Can you work these out from the model? Positions are in its coordinate system, mm. A direction names the side the tool comes from. Coordinates: 2 decimals unless noted, no trailing zeros. Write each loop counter-clockwise with the first axis right and the second up, starting at its lowest first coordinate (ties: lowest second). Pieces come first, ordered by that corner, then holes. Notation, with made-up numbers: M 70,60 L 122,60 A15 cw 122,79 Z; hole C 5,-23.75 d10. An arc over 180 degrees is marked long. Use one line per item in the form item = value. Start each with the question number.
```python
from build123d import *

# Parameters (mm, degrees)
SKETCH1_R           = 8.7376
BOSS_EXTRUDE1_DEPTH = 45.085
BOSS_EXTRUDE3_DEPTH = 4.516000112
FILLET2_R           = 5
BOSS_EXTRUDE4_START = 6.096
BOSS_EXTRUDE4_DEPTH = 6.096
CUT_EXTRUDE8_DEPTH  = 6.096
CUT_EXTRUDE10_DEPTH = 12.192
SKETCH23_R          = 1.5875
CUT_EXTRUDE11_DEPTH = 58.161632016
SKETCH24_R          = 3.175
SKETCH24_R_2        = 1.5875
CUT_EXTRUDE12_DEPTH = 54.671581882
CUT_EXTRUDE13_START = -1.27
SKETCH24_2_R        = 3.175
SKETCH24_2_R_2      = 1.5875
CUT_EXTRUDE13_DEPTH = 1.27
FILLET11_R          = 1.778
SKETCH25_R          = 2.5527
CUT_EXTRUDE14_DEPTH = 60.13111817


with BuildPart() as part:
    # Sketch1 → Boss-Extrude1 (new body)
    with BuildSketch(Plane.YZ):
        with Locations(Location((0, 0, 0), (0, 0, 270))):
            Circle(SKETCH1_R)
    extrude(amount=BOSS_EXTRUDE1_DEPTH)

    # Sketch10 → Boss-Extrude3 (add)
    with BuildSketch(Plane(origin=(0, 0, 0), x_dir=(0, -1, 0), z_dir=(-1, 0, 0))):
        with BuildLine():
            Line((0, 8.7376), (34.036, 8.7376))
            Line((34.036, 8.7376), (34.036, -8.7376))
            Line((34.036, -8.7376), (0, -8.7376))
            ThreePointArc((0, -8.7376), (8.7376, 0), (0, 8.7376))
        make_face()
    extrude(amount=-BOSS_EXTRUDE3_DEPTH)

    # Fillet2
    fillet2_edges = [part.edges().sort_by_distance(p)[0] for p in [
        (2.258000056, -34.036, 8.7376),
        (2.258000056, -34.036, -8.7376),
    ]]
    fillet(fillet2_edges, radius=FILLET2_R)

    # Sketch15 → Boss-Extrude4 (add)
    with BuildSketch(Plane.YZ.offset(4.516000112).offset(BOSS_EXTRUDE4_START)):
        with BuildLine():
            Line((-20.066, 5.472786999), (-29.036, 8.7376))
            ThreePointArc((-29.036, 8.7376), (-32.571533906, 7.273133906), (-34.036, 3.7376))
            Line((-34.036, 3.7376), (-34.036, -3.7376))
            ThreePointArc((-34.036, -3.7376), (-32.571533906, -7.273133906), (-29.036, -8.7376))
            Line((-29.036, -8.7376), (-20.066, -8.7376))
            Line((-20.066, -8.7376), (-20.066, 5.472786999))
        make_face()
    extrude(amount=-BOSS_EXTRUDE4_DEPTH)

    # Sketch21 → Cut-Extrude8 (cut)
    with BuildSketch(Plane.YZ.offset(10.612000112)):
        with BuildLine():
            Line((-20.701, -8.7376), (-20.066, -8.7376))
            Line((-20.066, -8.7376), (-20.066, 5.472786999))
            Line((-20.066, 5.472786999), (-20.662704814, 5.68996979))
            ThreePointArc((-20.662704814, 5.68996979), (-22.005444378, -1.520301887), (-20.701, -8.7376))
        make_face()
    extrude(amount=-CUT_EXTRUDE8_DEPTH, mode=Mode.SUBTRACT)

    # Sketch22 → Cut-Extrude10 (cut)
    with BuildSketch(Plane.YZ.offset(45.085)):
        with BuildLine():
            Line((-4.089715516, -2.794), (4.089715516, -2.794))
            ThreePointArc((4.089715516, -2.794), (4.953, 0), (4.089715516, 2.794))
            Line((4.089715516, 2.794), (-4.089715516, 2.794))
            ThreePointArc((-4.089715516, 2.794), (-4.953, 0), (-4.089715516, -2.794))
        make_face()
    extrude(amount=-CUT_EXTRUDE10_DEPTH, mode=Mode.SUBTRACT)

    # Sketch23 → Cut-Extrude11 (cut, through all)
    with BuildSketch(Plane.ZY):
        with Locations((0, -30.089710358)):
            Circle(SKETCH23_R)
        with Locations((0, -20.184348406)):
            Circle(SKETCH23_R)
    extrude(amount=-CUT_EXTRUDE11_DEPTH, mode=Mode.SUBTRACT)

    # Sketch24 → Cut-Extrude12 (cut, through all)
    with BuildSketch(Plane.YZ.offset(4.516000112)):
        with Locations((-20.184348406, 0)):
            Circle(SKETCH24_R)
        with Locations(Location((-20.184348406, 0, 0), (0, 0, 90))):
            Circle(SKETCH24_R_2, mode=Mode.SUBTRACT)
    extrude(amount=CUT_EXTRUDE12_DEPTH, mode=Mode.SUBTRACT)

    # Sketch24<2> → Cut-Extrude13 (cut)
    with BuildSketch(Plane.YZ.offset(4.516000112).offset(CUT_EXTRUDE13_START)):
        with Locations(Location((-20.184348406, 0, 0), (0, 0, 114.682734544))):
            Circle(SKETCH24_2_R)
        with Locations(Location((-20.184348406, 0, 0), (0, 0, 90))):
            Circle(SKETCH24_2_R_2, mode=Mode.SUBTRACT)
    extrude(amount=CUT_EXTRUDE13_DEPTH, mode=Mode.SUBTRACT)

    # Fillet11
    fillet11_edges = [part.edges().sort_by_distance(p)[0] for p in [
        (38.989, 4.089715516, 2.794),
        (38.989, 4.089715516, -2.794),
        (38.989, -4.089715516, -2.794),
        (38.989, -4.089715516, 2.794),
    ]]
    fillet(fillet11_edges, radius=FILLET11_R)

    # Sketch25 → Cut-Extrude14 (cut, through all)
    with BuildSketch(Plane(origin=(0, 0, -8.7376), x_dir=(1, 0, 0), z_dir=(0, 0, -1))):
        with Locations((7.068700112, 20.701)):
            Circle(SKETCH25_R)
    extrude(amount=-CUT_EXTRUDE14_DEPTH, mode=Mode.SUBTRACT)


solid = part.part
```
1) Suppose I cut it at A-A on z = 0. Please give me the cut outline in (x, y) (3 decimals).
2) Will these pins go through, and if not, where does the flat tip stop? pin 1 Ø1.5 at (x, z) = (34, -3) entering from -Y; pin 2 Ø7 at (y, z) = (-19.5, -0.5) entering from +X; pin 3 Ø1.5 at (x, y) = (29.5, -3) entering from +Z; pin 4 Ø1.9 at (y, z) = (-30.09, 0) entering from -X.
3) Please list where these lines run through material, in increasing order: line 1 (Y direction, x = 1.85, z = 0); line 2 (Y direction, x = 8, z = 0); line 3 (X direction, y = -19, z = 1.75).
4) Suppose I cut it at D-D on x = 13. Please give me the cut outline in (y, z).
5) Suppose I cut it at C-C on y = -11. Please give me the cut outline in (x, z).
6) Suppose I cut it at B-B on x = 40.5. Please give me the cut outline in (y, z).
7) If we mould it in two halves opening along X, with no side actions, what happens to faces 6 (the face through (7.125, -23.253, -5.711)), 7 (the face through (32.893, 0, 0)), 8 (the face through (38.9, -4.03, 2.47))? For each: +X half, -X half, draft (parallel to the pull), parting line (faces both ways), or undercut.
8) Which directions (+Z, -Z, +X, -X, +Y, -Y) give clear straight access to the entire face, cutting with the end or side of a thin tool? Please do faces 1 (the face through (5.23, -31.64, -0.34)), 2 (the face through (38.9, 4.03, -2.47)), 3 (the face through (5, -34.036, 0)), 4 (the face through (7.61, -25.72, 7.53)), 5 (the face through (10.612, -27, 0)).
Computed values:
q1.outline = M 0,-34.036 L 10.612,-34.036 L 10.612,-31.677 L 0,-31.677 Z; M 0,-28.502 L 10.612,-28.502 L 10.612,-23.359 L 3.246,-23.359 L 3.246,-21.772 L 0,-21.772 Z; M 0,-18.597 L 3.246,-18.597 L 3.246,-17.009 L 4.516,-17.009 L 4.516,-8.738 L 45.085,-8.738 L 45.085,-4.953 L 32.893,-4.953 L 32.893,4.953 L 45.085,4.953 L 45.085,8.738 L 0,8.738 Z
q2.pin_1 = -8.44
q2.pin_2 = 10.61
q2.pin_3 = 8.44
q2.pin_4 = through
q3.line_1 = -34.04 to -31.68, -28.5 to -21.77, -18.6 to 8.74
q3.line_2 = -34.04 to -31.68, -28.5 to -23.36, -8.74 to 8.74
q3.line_3 = 0 to 3.25
q4.outline = C 0,0 d17.48
q5.outline = M 0,-8.74 L 4.52,-8.74 L 4.52,8.74 L 0,8.74 Z
q6.outline = C 0,0 d17.48; hole M -4.69,-1.58 A1.78 ccw -3.01,-2.79 L 3.01,-2.79 A1.78 ccw 4.69,-1.58 A4.95 ccw 4.69,1.58 A1.78 ccw 3.01,2.79 L -3.01,2.79 A1.78 ccw -4.69,1.58 A4.95 ccw Z
q7.face_6 = undercut
q7.face_7 = +X half
q7.face_8 = draft
q8.face_1 = +X, -X
q8.face_2 = +X
q8.face_3 = +Z, -Z, +X, -X, -Y
q8.face_4 = +Z, +X
q8.face_5 = +Z, -Z, +X, -Y
